from build123d import *

# Parameters (mm, degrees)
EXTRUDE_1_DEPTH     = 90
SKETCH_2_R          = 1.75
CUT_EXTRUDE_1_DEPTH = 130.002266823
SKETCH_3_R          = 4
SKETCH_3_W          = 25
SKETCH_3_H          = 39
SKETCH_3_W_2        = 10.5
SKETCH_3_H_2        = 10
SKETCH_3_W_3        = 22
SKETCH_3_H_3        = 11
SKETCH_3_W_4        = 11
SKETCH_3_W_5        = 14
SKETCH_3_H_4        = 9
SKETCH_3_W_6        = 9.5
SKETCH_3_H_5        = 42
SKETCH_3_W_7        = 8
SKETCH_3_H_6        = 16
SKETCH_3_W_8        = 19
SKETCH_3_H_7        = 23
CUT_EXTRUDE_2_DEPTH = 130.002266823
CUT_EXTRUDE_3_REACH = 133.002
CUT_EXTRUDE_START   = -2
CUT_EXTRUDE_4_DEPTH = 1.5
SKETCH_6_W          = 90
SKETCH_6_H          = 5
EXTRUDE_2_DEPTH     = 0.5
SKETCH_7_R          = 2.65
CUT_EXTRUDE_5_DEPTH = 118.968449984
CUT_EXTRUDE_6_REACH = 123.968
CUT_EXTRUDE_START_2 = -4
SKETCH_8_R          = 5
SKETCH_9_R          = 3.5
EXTRUDE_3_DEPTH     = 2.5
SKETCH_10_R         = 1.75
CUT_EXTRUDE_7_DEPTH = 130.354890357
CUT_EXTRUDE_8_REACH = 141.002
CUT_EXTRUDE_START_3 = -10
SKETCH_11_W         = 28.5
SKETCH_11_H         = 18
SKETCH_12_W         = 10
SKETCH_12_H         = 98.345155262
SKETCH_12_H_2       = 101.038352977
CUT_EXTRUDE_9_DEPTH = 129.917968218


with BuildPart() as part:
    # 草图1 → 凸台-拉伸1 (new body)
    with BuildSketch(Plane(origin=(0, 0, 0), x_dir=(0, 0, -1), z_dir=(1, 0, 0))):
        Polygon((0, 0), (0, 76), (-14.849242405, 90.849242405), (-16.970562748, 88.727922061), (-5, 0), align=None)
    extrude(amount=EXTRUDE_1_DEPTH)

    # 草图2 → 切除-拉伸1 (cut, through all)
    with BuildSketch(Plane(origin=(0, 0, 0), x_dir=(-1, 0, 0), z_dir=(0, 0, -1))):
        with Locations((-75, 64)):
            Circle(SKETCH_2_R)
        with Locations((-15, 64)):
            Circle(SKETCH_2_R)
        with Locations((-15, 14)):
            Circle(SKETCH_2_R)
        with Locations((-75, 14)):
            Circle(SKETCH_2_R)
    extrude(amount=-CUT_EXTRUDE_1_DEPTH, mode=Mode.SUBTRACT)

    # 草图3 → 切除-拉伸2 (cut, through all)
    with BuildSketch(Plane(origin=(0, 0, 0), x_dir=(-1, 0, 0), z_dir=(0, 0, -1))):
        with Locations((-74, 33.5)):
            Circle(SKETCH_3_R)
        with Locations((-26, 38.5)):
            Rectangle(SKETCH_3_W, SKETCH_3_H)
        with Locations((-25.75, 14)):
            Rectangle(SKETCH_3_W_2, SKETCH_3_H_2)
        with Locations((-31, 61.5)):
            Rectangle(SKETCH_3_W_3, SKETCH_3_H_3)
        with Locations((-43.5, 60.5)):
            Rectangle(SKETCH_3_W_4, SKETCH_3_H_3)
        with Locations((-63.5, 62.5)):
            Rectangle(SKETCH_3_W_5, SKETCH_3_H_4)
        with Locations((-85.25, 34)):
            Rectangle(SKETCH_3_W_6, SKETCH_3_H_5)
        with Locations((-66.5, 21)):
            Rectangle(SKETCH_3_W_7, SKETCH_3_H_6)
        with Locations((-56.5, 42)):
            Rectangle(SKETCH_3_W_8, SKETCH_3_H_7)
    extrude(amount=-CUT_EXTRUDE_2_DEPTH, mode=Mode.SUBTRACT)

    # 切除-拉伸3: up to this plane
    cut_extrude_3_end = Plane(origin=(90, 88.727922061, 16.970562748), z_dir=(0, 0.13370183830700452, -0.9910216034140364))
    # 草图4 → 切除-拉伸3 (cut, up to the surface)
    with BuildSketch(Plane(origin=(0, 0, 0), x_dir=(-1, 0, 0), z_dir=(0, 0, -1)).offset(CUT_EXTRUDE_START), mode=Mode.PRIVATE) as cut_extrude_3_sk1:
        Polygon((-75, 60.651368439), (-72.1, 62.325684219), (-72.1, 65.674315781), (-75, 67.348631561), (-77.9, 65.674315781), (-77.9, 62.325684219), align=None)
    cut_extrude_3_tool1 = split(extrude(cut_extrude_3_sk1.sketch, amount=-CUT_EXTRUDE_3_REACH, mode=Mode.PRIVATE), bisect_by=cut_extrude_3_end, keep=Keep.BOTH, mode=Mode.PRIVATE)
    add(cut_extrude_3_tool1.solids().sort_by_distance((75, 64, 2))[0], mode=Mode.SUBTRACT)
    # 草图4 → 切除-拉伸3 (cut, up to the surface)
    with BuildSketch(Plane(origin=(0, 0, 0), x_dir=(-1, 0, 0), z_dir=(0, 0, -1)).offset(CUT_EXTRUDE_START), mode=Mode.PRIVATE) as cut_extrude_3_sk2:
        Polygon((-15, 60.651368439), (-12.1, 62.325684219), (-12.1, 65.674315781), (-15, 67.348631561), (-17.9, 65.674315781), (-17.9, 62.325684219), align=None)
    cut_extrude_3_tool2 = split(extrude(cut_extrude_3_sk2.sketch, amount=-CUT_EXTRUDE_3_REACH, mode=Mode.PRIVATE), bisect_by=cut_extrude_3_end, keep=Keep.BOTH, mode=Mode.PRIVATE)
    add(cut_extrude_3_tool2.solids().sort_by_distance((15, 64, 2))[0], mode=Mode.SUBTRACT)
    # 草图4 → 切除-拉伸3 (cut, up to the surface)
    with BuildSketch(Plane(origin=(0, 0, 0), x_dir=(-1, 0, 0), z_dir=(0, 0, -1)).offset(CUT_EXTRUDE_START), mode=Mode.PRIVATE) as cut_extrude_3_sk3:
        Polygon((-15, 10.651368439), (-12.1, 12.325684219), (-12.1, 15.674315781), (-15, 17.348631561), (-17.9, 15.674315781), (-17.9, 12.325684219), align=None)
    cut_extrude_3_tool3 = split(extrude(cut_extrude_3_sk3.sketch, amount=-CUT_EXTRUDE_3_REACH, mode=Mode.PRIVATE), bisect_by=cut_extrude_3_end, keep=Keep.BOTH, mode=Mode.PRIVATE)
    add(cut_extrude_3_tool3.solids().sort_by_distance((15, 14, 2))[0], mode=Mode.SUBTRACT)
    # 草图4 → 切除-拉伸3 (cut, up to the surface)
    with BuildSketch(Plane(origin=(0, 0, 0), x_dir=(-1, 0, 0), z_dir=(0, 0, -1)).offset(CUT_EXTRUDE_START), mode=Mode.PRIVATE) as cut_extrude_3_sk4:
        Polygon((-75, 10.651368439), (-72.1, 12.325684219), (-72.1, 15.674315781), (-75, 17.348631561), (-77.9, 15.674315781), (-77.9, 12.325684219), align=None)
    cut_extrude_3_tool4 = split(extrude(cut_extrude_3_sk4.sketch, amount=-CUT_EXTRUDE_3_REACH, mode=Mode.PRIVATE), bisect_by=cut_extrude_3_end, keep=Keep.BOTH, mode=Mode.PRIVATE)
    add(cut_extrude_3_tool4.solids().sort_by_distance((75, 14, 2))[0], mode=Mode.SUBTRACT)

    # 草图5 → 切除-拉伸4 (cut)
    with BuildSketch(Plane(origin=(0, 0, 0), x_dir=(-1, 0, 0), z_dir=(0, 0, -1))):
        Polygon((-70.5, 20), (-70.5, 29), (-62.5, 29), (-62.5, 0), (-49.5, 0), (-49.5, 30.5), (-66, 30.5), (-66, 53.5), (-80.5, 53.5), (-80.5, 20), align=None)
    extrude(amount=-CUT_EXTRUDE_4_DEPTH, mode=Mode.SUBTRACT)

    # 草图6 → 凸台-拉伸2 (add)
    with BuildSketch(Plane(origin=(0, 38, -38), x_dir=(1, 0, 0), z_dir=(0, 0.7071067811865482, -0.7071067811865468))):
        with Locations((45, -64.74011537)):
            Rectangle(SKETCH_6_W, SKETCH_6_H)
    extrude(amount=EXTRUDE_2_DEPTH)

    # 草图7 → 切除-拉伸5 (cut, through all)
    with BuildSketch(Plane(origin=(0, 38.353553391, -38.353553391), x_dir=(1, 0, 0), z_dir=(0, 0.7071067811865489, -0.7071067811865461))):
        with Locations(Location((20, -64.74011537, 0), (0, 0, 270))):
            Circle(SKETCH_7_R)
        with Locations(Location((70, -64.74011537, 0), (0, 0, 270))):
            Circle(SKETCH_7_R)
    extrude(amount=-CUT_EXTRUDE_5_DEPTH, mode=Mode.SUBTRACT)

    # 切除-拉伸6: up to this plane
    cut_extrude_6_end = Plane(origin=(90, 88.727922061, 16.970562748), z_dir=(0, 0.13370183830700452, -0.9910216034140364))
    # 草图8 → 切除-拉伸6 (cut, up to the surface)
    with BuildSketch(Plane(origin=(0, 38.353553391, -38.353553391), x_dir=(1, 0, 0), z_dir=(0, 0.7071067811865489, -0.7071067811865461)).offset(CUT_EXTRUDE_START_2), mode=Mode.PRIVATE) as cut_extrude_6_sk1:
        with Locations(Location((20, -64.74011537, 0), (0, 0, 270))):
            Circle(SKETCH_8_R)
    cut_extrude_6_tool1 = split(extrude(cut_extrude_6_sk1.sketch, amount=-CUT_EXTRUDE_6_REACH, mode=Mode.PRIVATE), bisect_by=cut_extrude_6_end, keep=Keep.BOTH, mode=Mode.PRIVATE)
    add(cut_extrude_6_tool1.solids().sort_by_distance((20, 81.303301, 10.253048))[0], mode=Mode.SUBTRACT)
    # 草图8 → 切除-拉伸6 (cut, up to the surface)
    with BuildSketch(Plane(origin=(0, 38.353553391, -38.353553391), x_dir=(1, 0, 0), z_dir=(0, 0.7071067811865489, -0.7071067811865461)).offset(CUT_EXTRUDE_START_2), mode=Mode.PRIVATE) as cut_extrude_6_sk2:
        with Locations(Location((70, -64.74011537, 0), (0, 0, 270))):
            Circle(SKETCH_8_R)
    cut_extrude_6_tool2 = split(extrude(cut_extrude_6_sk2.sketch, amount=-CUT_EXTRUDE_6_REACH, mode=Mode.PRIVATE), bisect_by=cut_extrude_6_end, keep=Keep.BOTH, mode=Mode.PRIVATE)
    add(cut_extrude_6_tool2.solids().sort_by_distance((70, 81.303301, 10.253048))[0], mode=Mode.SUBTRACT)

    # 草图9 → 凸台-拉伸3 (add)
    with BuildSketch(Plane(origin=(0, 0, 0), x_dir=(-1, 0, 0), z_dir=(0, 0, -1))):
        with Locations(Location((-75, 64, 0), (0, 0, 180))):
            Circle(SKETCH_9_R)
        with Locations(Location((-15, 64, 0), (0, 0, 180))):
            Circle(SKETCH_9_R)
        with Locations(Location((-15, 14, 0), (0, 0, 180))):
            Circle(SKETCH_9_R)
        with Locations(Location((-75, 14, 0), (0, 0, 180))):
            Circle(SKETCH_9_R)
    extrude(amount=EXTRUDE_3_DEPTH)

    # 草图10 → 切除-拉伸7 (cut, through all)
    with BuildSketch(Plane(origin=(0, 0, -2.5), x_dir=(-1, 0, 0), z_dir=(0, 0, -1))):
        with Locations((-75, 14)):
            Circle(SKETCH_10_R)
        with Locations((-15, 14)):
            Circle(SKETCH_10_R)
        with Locations((-15, 64)):
            Circle(SKETCH_10_R)
        with Locations((-75, 64)):
            Circle(SKETCH_10_R)
    extrude(amount=-CUT_EXTRUDE_7_DEPTH, mode=Mode.SUBTRACT)

    # 草图11 → 切除-拉伸8 (cut, up to next)
    with BuildSketch(Plane(origin=(0, 0, 0), x_dir=(-1, 0, 0), z_dir=(0, 0, -1)).offset(CUT_EXTRUDE_START_3), mode=Mode.PRIVATE) as cut_extrude_8_sk1:
        with Locations((-27.75, 65)):
            Rectangle(SKETCH_11_W, SKETCH_11_H)
    cut_extrude_8_tool1 = extrude(cut_extrude_8_sk1.sketch, amount=-CUT_EXTRUDE_8_REACH, mode=Mode.PRIVATE) & part.part
    add(cut_extrude_8_tool1.solids().sort_by_distance((27.75, 65, 10))[0], mode=Mode.SUBTRACT)

    # 草图12 → 切除-拉伸9 (cut, through all)
    with BuildSketch(Plane(origin=(0, -0.662507051, 4.910619092), x_dir=(1, 0, 0), z_dir=(0, -0.13370183830700455, 0.9910216034140364))):
        with Locations((5, 45.332571267)):
            Rectangle(SKETCH_12_W, SKETCH_12_H)
        with Locations((85, 43.98597241)):
            Rectangle(SKETCH_12_W, SKETCH_12_H_2)
    extrude(amount=-CUT_EXTRUDE_9_DEPTH, mode=Mode.SUBTRACT)


solid = part.part
Geometry check sheet. Reference: the model listing, model coordinates, mm. A direction names the side the tool comes from. Coordinates: 2 decimals unless noted, no trailing zeros. Order: outer loops, then holes, each group sorted by start corner. A loop starts at its lowest first (then second) coordinate and runs counter-clockwise, first axis right, second up. Notation, with made-up numbers: M 3.25,34 L 34.25,34 A24 cw 34.25,71 Z; hole C -32,14.5 d11. An arc over 180 degrees is marked long. Use CSV: the item, a comma, the result in double quotes.
Item 1: Thickness scan on line 1 along X through (y, z) = (60, 1.25); line 2 along X through (y, z) = (64, -1.35); line 3 along X through (y, z) = (40, 1.25). Record the ranges inside material, lowest first.
Returned:
line 1,"x = 10 to 20, 49 to 56.5, 70.5 to 80"
line 2,"x = 11.5 to 13.25, 16.75 to 18.5, 71.5 to 73.25, 76.75 to 78.5"
line 3,"x = 10 to 13.5, 38.5 to 47"
Item 2: Cross-section at C-C on z = 3.5. Give the number of separate pieces and of enclosed holes in the cut face, then the cut area to 3 significant figures.
Returned:
separate pieces,"1"
enclosed holes,"9"
area,"3,340 mm2"
Item 3: Tool access check on faces 4 (the flat face through (13, 15, -2.5)), 5 (the flat face through (67, 13, 3)), 6 (the flat face through (13.75, 12.56, 2)), 7 (the cylindrical face through (78.233, 15.341, -1.232)). Record the directions out of +Z, -Z, +X, -X, +Y, -Y that give a thin tool (end or side, any length) a straight path to the whole face; none if there is none.
Returned:
face 4,"-Z, +X, -X, +Y, -Y"
face 5,"+Z, -Z"
face 6,"+Z"
face 7,"-Z"
Item 4: Cross-section at B-B on y = 33.5. Record the cut outline in (x, z).
Returned:
outline,"M 10,0 L 13.5,0 L 13.5,9.52 L 10,9.52 Z; M 38.5,0 L 47,0 L 47,9.52 L 38.5,9.52 Z; M 66,1.5 L 70,1.5 L 70,9.52 L 66,9.52 Z; M 78,1.5 L 80,1.5 L 80,9.52 L 78,9.52 Z"
Item 5: Mould release check, pull along Y, two halves, no side actions. Record for faces 1 (the flat face through (13.5, 70, 12)), 2 (the flat face through (76.43, 66.523, 7.959)), 3 (the flat face through (44.662, 84.107, 7.4)): pulls with the +Y half, pulls with the -Y half, needs draft (parallel to the pull), parting line crosses it, or undercut.
Returned:
face 1,"needs draft"
face 2,"undercut"
face 3,"pulls with the +Y half"
Item 6: Cross-section at A-A on x = 52. Record the cut outline in (y, z), then the cut area to 3 significant figures.
Returned:
outline,"M 0,1.5 L 30.5,1.5 L 30.5,9.11 L 0,5 Z; M 53.5,0 L 76,0 L 82.01,6.01 L 82.36,5.66 L 85.9,9.19 L 85.55,9.55 L 90.85,14.85 L 88.73,16.97 L 53.5,12.22 Z"
area,"610 mm2"
Item 7: Gauge pin test, flat ends, axial feed: pin 1 Ø5.5 at (x, z) = (65, 3.5) entering from +Y; pin 2 Ø4 at (x, z) = (33.5, 4.5) entering from +Y; pin 3 Ø4 at (x, z) = (73, 3) entering from +Y; pin 4 Ø3 at (x, y) = (75, 14) entering from -Z. Record the tip position at first contact, or that the pin passes through.
Returned:
pin 1,"stops at y = 82.96"
pin 2,"stops at y = 83.21"
pin 3,"stops at y = 81"
pin 4,"passes through"
